Autodesk Inventor part; units mm, degrees
ref_plane "Work Plane1" through (0, -4, 0) normal (0, -1, 0) x (1, 0, 0)
ref_plane "YZ Plane" through (0, 0, 0) normal (1, 0, 0) x (0, 1, 0)
ref_plane "XZ Plane" through (0, 0, 0) normal (0, 1, 0) x (-1, 0, 0)
sketch "Sketch1" plane through (0, 0, 0) normal (0, 1, 0) x (-1, 0, 0)
  circle A0 centre (0, 0) radius 24
  dimension "d0" = 48
extrude "Extrusion1" add sketch "Sketch1" against normal blind 8
fillet "Fillet1" radius 4 2 edges at (24, 0, 0) (24, -8, 0)
sketch "Sketch2" plane through (0, -8, 0) normal (0, -1, 0) x (1, 0, 0)
  circle A0 centre (0, 0) radius 12
  line L0 (-7.3581, 9.4794) -> (-3.0473, 5.1686)
  arc A1 (-1.5, 5.8095) -> (-3.0473, 5.1686) centre (0, 0) ccw
  line L1 (-1.5, 5.8095) -> (-1.5, 11.9059)
  arc A2 (-1.5, 11.9059) -> (-7.3581, 9.4794) centre (0, 0) ccw
  line L2 (3.0473, 5.1686) -> (7.3581, 9.4794)
  arc A3 (7.3581, 9.4794) -> (1.5, 11.9059) centre (0, 0) ccw
  line L3 (1.5, 11.9059) -> (1.5, 5.8095)
  arc A4 (3.0473, 5.1686) -> (1.5, 5.8095) centre (0, 0) ccw
  line L4 (9.4794, 7.3581) -> (5.1686, 3.0473)
  arc A5 (5.8095, 1.5) -> (5.1686, 3.0473) centre (0, 0) ccw
  line L5 (5.8095, 1.5) -> (11.9059, 1.5)
  arc A6 (11.9059, 1.5) -> (9.4794, 7.3581) centre (0, 0) ccw
  line L6 (11.9059, -1.5) -> (5.8095, -1.5)
  arc A7 (5.1686, -3.0473) -> (5.8095, -1.5) centre (0, 0) ccw
  line L7 (5.1686, -3.0473) -> (9.4794, -7.3581)
  arc A8 (9.4794, -7.3581) -> (11.9059, -1.5) centre (0, 0) ccw
  line L8 (7.3581, -9.4794) -> (3.0473, -5.1686)
  arc A9 (1.5, -5.8095) -> (3.0473, -5.1686) centre (0, 0) ccw
  line L9 (1.5, -5.8095) -> (1.5, -11.9059)
  arc A10 (1.5, -11.9059) -> (7.3581, -9.4794) centre (0, 0) ccw
  line L10 (-3.0473, -5.1686) -> (-7.3581, -9.4794)
  arc A11 (-7.3581, -9.4794) -> (-1.5, -11.9059) centre (0, 0) ccw
  line L11 (-1.5, -11.9059) -> (-1.5, -5.8095)
  arc A12 (-3.0473, -5.1686) -> (-1.5, -5.8095) centre (0, 0) ccw
  line L12 (-9.4794, -7.3581) -> (-5.1686, -3.0473)
  arc A13 (-5.8095, -1.5) -> (-5.1686, -3.0473) centre (0, 0) ccw
  line L13 (-5.8095, -1.5) -> (-11.9059, -1.5)
  arc A14 (-11.9059, -1.5) -> (-9.4794, -7.3581) centre (0, 0) ccw
  line L14 (-5.1686, 3.0473) -> (-9.4794, 7.3581)
  arc A15 (-9.4794, 7.3581) -> (-11.9059, 1.5) centre (0, 0) ccw
  line L15 (-11.9059, 1.5) -> (-5.8095, 1.5)
  arc A16 (-5.1686, 3.0473) -> (-5.8095, 1.5) centre (0, 0) ccw
  circle A17 centre (0, 0) radius 6
  circle A18 centre (0, 0) radius 2.1
  point P0 (-6, 0)
extrude "Extrusion2" cut sketch "Sketch2" against normal blind 0.5 contours L5 A5 L4 A0 | A0 L7 A7 L6 | L2 A4 L3 A0 | A0 L9 A9 L8 | L1 A1 L0 A0 | A0 L10 A12 L11 | L14 A16 L15 A0 | A0 L13 A13 L12
sketch "Sketch3" plane through (0, -8, 0) normal (0, -1, 0) x (1, 0, 0)
  arc A0 (3.0473, 5.1686) -> (1.5, 5.8095) centre (0, 0) ccw
  circle A1 centre (0, 0) radius 6
extrude "Extrusion3" add sketch "Sketch3" along normal blind 3.5
ref_plane "Work Plane1" through (0, -4, 0) normal (0, -1, 0) x (1, 0, 0)
mirror "Mirror1" about plane through (0, -4, 0) normal (0, -1, 0) of "Extrusion2", "Extrusion3"
sketch "Sketch4" plane through (0, -11.5, 0) normal (0, -1, 0) x (1, 0, 0)
  point P0 (0, 0)
hole "Hole1" at (0, -11.5, 0) direction (0, 1, 0) diameter 4.5 end through all
properties part number "13-0003" material "Polystyrene, High Impact"
The listing builds one solid part. Answer for the finished solid, in the listing's coordinates (mm). A direction names the side the tool comes from. Give positions to 0.01 mm unless a question says otherwise; leave off trailing zeros. Loops run counter-clockwise (first coordinate to the right, second up) from the corner with the lowest first, then second, coordinate; pieces in that order, holes last. Notation, with made-up numbers: (38, -8) - (47, -8) arc R26 cw to (47, 16) - close; hole circle Ø5 at (36.25, 75.25). An arc over 180 degrees is marked (long way). Use one line per item in the form item = value.
1. The mould has two halves that part along X. Classify faces 1 (the face through (5, 0, -4)), 2 (the face through (4.63, -7.75, 11.07)), 3 (the face through (-2.061, -9.726, -5.635)): pulls with the +X half, pulls with the -X half, needs draft (parallel to the pull), parting line crosses it, or undercut.
Calculated:
face_1 = needs draft
face_2 = undercut
face_3 = parting line crosses it
2. Section B-B on y = -1.25 is taken. Give the vertices of the cut face in (x, z), then the cut area to 3 significant figures.
Calculated:
outline = circle Ø45.81 at (0, 0); hole circle Ø4.5 at (0, 0)
area = 1,630 mm^2
3. Section C-C on y = -6.25 is taken. Give the vertices of the cut face in (x, z).
Calculated:
outline = circle Ø46.61 at (0, 0); hole circle Ø4.5 at (0, 0)
4. Section D-D on y = -10 is taken. Give the vertices of the cut face in (x, z).
Calculated:
outline = (1.5, 5.81) arc R6 ccw (long way) to (3.05, 5.17) arc R6 ccw to start; hole circle Ø4.5 at (0, 0)
5. Find the intervals of material crossed by line 1 along X through (y, z) = (0.25, 0); line 2 along Z through (x, y) = (1, 2.5); line 3 along Y through (x, z) = (0, -14), in increasing order. Write a range as [from, to].
Calculated:
line_1 = [-6, -2.25], [2.25, 6]
line_2 = [-5.92, -2.02], [2.02, 5.92]
line_3 = [-8, 0]
6. Given pin 1 Ø6 at (y, z) = (-10, -1.5) entering from +X; pin 2 Ø4 at (x, z) = (-11.5, 11) entering from +Y; pin 3 Ø4.5 at (x, z) = (5.5, -9) entering from -Y, each flat-ended and moving along its own axis, determine where each tip first touches the part or whether it passes through.
Calculated:
pin_1 = 22.6
pin_2 = 0
pin_3 = -8
7. Which of the six approach directions +Z, -Z, +X, -X, +Y, -Y give full straight-line access (tool end or side, diameter ignored) to faces 4 (the face through (-2.53, 1.73, -5.44)), 5 (the face through (5, -8, -4))?
Calculated:
face_4 = +Y
face_5 = -Y
